Here's how the part is built. I have some questions about the finished solid (model axes, mm). A direction names the side the tool comes from. Round coordinates to 2 decimals unless told otherwise and drop trailing zeros. Write each loop counter-clockwise with the first axis right and the second up, starting at its lowest first coordinate (ties: lowest second). Pieces come first, ordered by that corner, then holes. Notation, with made-up numbers: (74, 10) - (122, 10) arc R34 cw to (122, 40) - close; hole circle Ø8 at (-38, 70.25). An arc over 180 degrees is marked (long way). One line per item, written item: value. Start each with the question number.
Item 1: For P1, Ø6, axis at x = 201.5, z = 33, coming from the +Y side; P2, Ø4, axis at x = 74, y = -201.5, coming from the +Z side; P3, Ø1, axis at x = 82, z = 121.5, coming from the -Y side, each with a flat end and sliding along its axis, tell me the tip position at first contact or that it passes through.
Item 2: For faces 1 (the face through (179, -350, 9)), 2 (the face through (179, -18, 99)), which set-ups out of +Z, -Z, +X, -X, +Y, -Y let a thin tool reach every point of the face, with its end or its side?
Item 3: Imagine slicing it at A-A, the plane y = -317. Please give me the cut outline in (x, z).
Item 4: Imagine slicing it at C-C, the plane z = 167.5. Please give me the cut outline in (x, y).
Item 5: If I drill on line 1 (Y direction, x = 257.5, z = 33); line 2 (Z direction, x = 49, y = -332.5), over which ranges is the centre line in solid material (lowest first)?
Item 6: Imagine slicing it at B-B, the plane x = 248. Please give me the cut outline in (y, z).
```python
from build123d import *

# Parameters (mm, degrees)
F0_W     = 37.1829867363
F0_H     = 34.0256392956
F1_DEPTH = 350
F2_DEPTH = 400
F3_DEPTH = 180
F4_T     = -18
F5_DEPTH = 36
F6_R     = 2
F7_R     = 2
F8_R     = 2


with BuildPart() as f1:
    # F0 (on Front) → F1 (new body)
    with BuildSketch(Plane.XZ):
        with Locations((18.5914933681, 17.0128196478)):
            Rectangle(F0_W, F0_H)
    extrude(amount=F1_DEPTH)

    # F2 (add): a face of the model
    f2_faces = [f1.faces().sort_by_distance(p)[0] for p in [
        (0, -175, 17.0128196478),
    ]]
    extrude(f2_faces, amount=-F2_DEPTH)

    # F3 (add): a face of the model
    f3_faces = [f1.faces().sort_by_distance(p)[0] for p in [
        (200, -175, 0),
    ]]
    extrude(f3_faces, amount=-F3_DEPTH)

    # F4
    f4_openings = [f1.faces().sort_by_distance(p)[0] for p in [
        (0, -175, 90),
        (200, -350, 90),
        (200, -175, 180),
        (400, -175, 90),
    ]]
    offset(amount=F4_T, openings=f4_openings)

    # F5 (cut): a face of the model
    f5_faces = [f1.faces().sort_by_distance(p)[0] for p in [
        (400, -9, 176.0642662692),
    ]]
    extrude(f5_faces, amount=-F5_DEPTH, mode=Mode.SUBTRACT)

    # F6
    f6_edges = [f1.edges().sort_by_distance(p)[0] for p in [
        (182, -350, 0),
    ]]
    fillet(f6_edges, radius=F6_R)

    # F7
    f7_edges = [f1.edges().sort_by_distance(p)[0] for p in [
        (364, -350, 10),
        (0, -350, 10),
    ]]
    fillet(f7_edges, radius=F7_R)

    # F8
    f8_edges = [f1.edges().sort_by_distance(p)[0] for p in [
        (182, -350, 18),
    ]]
    fillet(f8_edges, radius=F8_R)


solid = f1.part
```
Values follow:
1. P1: stops at y = 0
1. P2: stops at z = 18
1. P3: stops at y = -18
2. face 1: +Z, -Z, +X, -X, -Y
2. face 2: +Z, +X, -X, -Y
3. outline: (0, 2) arc R2 ccw to (2, 0) - (362, 0) arc R2 ccw to (364, 2) - (364, 16) arc R2 ccw to (362, 18) - (2, 18) arc R2 ccw to (0, 16) - close
4. outline: (0, -18) - (364, -18) - (364, 0) - (0, 0) - close
5. line 1: y = -18 to 0
5. line 2: z = 0 to 18
6. outline: (-350, 2) arc R2 ccw to (-348, 0) - (0, 0) - (0, 180) - (-18, 180) - (-18, 18) - (-348, 18) arc R2 ccw to (-350, 16) - close
